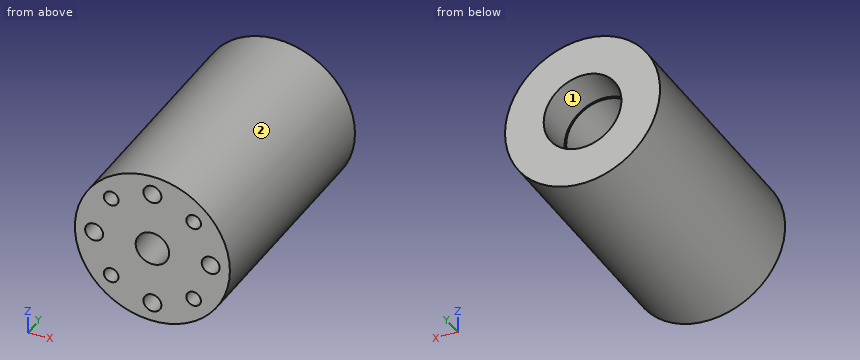
```python
from build123d import *

# Parameters (mm, degrees)
CUT_EXTRUDE2_START = -22.2
SKETCH4_R          = 1.1
SKETCH4_R_2        = 0.9
CUT_EXTRUDE2_DEPTH = 8


with BuildPart() as part:
    # Sketch1 → Revolve1 (revolve)
    with BuildSketch(Plane.XY):
        Polygon((4.762351203, 30), (4.762351203, 25), (4.559151203, 25), (2.05, 0), (9.5, -0.008522661), (9.5, 30), align=None)
    revolve(axis=Axis((0, 0, 0), (0, 1, 0)))

    # Sketch4 → Cut-Extrude2 (cut)
    with BuildSketch(Plane(origin=(0, 30, 0), x_dir=(1, 0, 0), z_dir=(0, 1, 0)).offset(CUT_EXTRUDE2_START)):
        with Locations(Location((0, 7.145, 0), (0, 0, 180))):
            Circle(SKETCH4_R)
        with Locations(Location((7.145, 0, 0), (0, 0, 180))):
            Circle(SKETCH4_R)
        with Locations(Location((0, -7.145, 0), (0, 0, 180))):
            Circle(SKETCH4_R)
        with Locations(Location((-7.145, 0, 0), (0, 0, 180))):
            Circle(SKETCH4_R)
        with Locations(Location((5.052277952, 5.052277952, 0), (0, 0, 180))):
            Circle(SKETCH4_R_2)
        with Locations(Location((5.052277952, -5.052277952, 0), (0, 0, 180))):
            Circle(SKETCH4_R_2)
        with Locations(Location((-5.052277952, -5.052277952, 0), (0, 0, 180))):
            Circle(SKETCH4_R_2)
        with Locations(Location((-5.052277952, 5.052277952, 0), (0, 0, 180))):
            Circle(SKETCH4_R_2)
    extrude(amount=-CUT_EXTRUDE2_DEPTH, mode=Mode.SUBTRACT)


solid = part.part
```
Check sheet for the modelled part. Datum: model origin and axes. Units: mm. Face numbers are marked on the shaded views. Round coordinates to 2 decimals unless told otherwise and drop trailing zeros. Loops run counter-clockwise (first coordinate to the right, second up) from the corner with the lowest first, then second, coordinate; pieces in that order, holes last. Notation, with made-up numbers: (-7.75, -9.5) -> (29.25, -9.5) arc R22 ccw to (29.25, 5.5) -> close; hole circle Ø4 at (4, -28.75). An arc over 180 degrees is marked (long way). Write item = value, one per line. Start each with the question number.
1) Sectioned sample at D-D, the plane y = 10. Record the cut outline in (x, z), plus the area to 3 significant figures.
2) Sectioned sample at C-C, the plane y = 20.5. Record the cut outline in (x, z) (1 decimal), plus the area to 3 significant figures.
3) Release check for a two-part mould opening along X. For the marked faces 1 and 2 record: released by +X, released by -X, zero draft, split by the parting line, or undercut.
4) Gauge pin test, flat ends, axial feed: pin 1 Ø2.5 at (x, z) = (-0.5, -7) entering from -Y; pin 2 Ø5 at (y, z) = (18, 3) entering from +X; pin 3 Ø1.6 at (x, z) = (5.05, 5.05) entering from -Y; pin 4 Ø5 at (x, y) = (-4.5, 24) entering from -Z. Record the tip position at first contact, or that the pin passes through.
5) Thickness scan on probe 1 along Z at (x, y) = (0, 5) (3 decimals); probe 2 along X at (y, z) = (6.25, 0) (3 decimals); probe 3 along Y at (x, z) = (-1, 6.25). Record the ranges inside material, lowest first.
6) Sectioned sample at B-B, the plane x = 0. Record the cut outline in (y, z) (3 decimals).
7) Sectioned sample at A-A, the plane z = 0. Record the cut outline in (x, y) (3 decimals).
Results are:
q1.outline = circle Ø19 at (0, 0); hole circle Ø6.11 at (0, 0)
q1.area = 254 mm^2
q2.outline = circle Ø19 at (0, 0); hole circle Ø8.2 at (0, 0)
q2.area = 231 mm^2
q3.face_1 = undercut
q3.face_2 = split by the parting line
q4.pin_1 = -0.01
q4.pin_2 = 9.49
q4.pin_3 = 7.8
q4.pin_4 = -9.29
q5.probe_1 = -9.5 to -8.245, -6.045 to -2.552, 2.552 to 6.045, 8.245 to 9.5
q5.probe_2 = -9.5 to -8.245, -6.045 to -2.677, 2.677 to 6.045, 8.245 to 9.5
q5.probe_3 = 0 to 30
q6.outline = (-0.009, -9.5) -> (30, -9.5) -> (30, -4.762) -> (25, -4.762) -> (25, -4.559) -> (0, -2.05) -> (-0.005, -6.045) -> (7.8, -6.045) -> (7.8, -8.245) -> (-0.007, -8.245) -> close; (-0.009, 9.5) -> (-0.007, 8.245) -> (7.8, 8.245) -> (7.8, 6.045) -> (-0.005, 6.045) -> (0, 2.05) -> (25, 4.559) -> (25, 4.762) -> (30, 4.762) -> (30, 9.5) -> close
q7.outline = (-9.5, -0.009) -> (-8.245, -0.007) -> (-8.245, 7.8) -> (-6.045, 7.8) -> (-6.045, -0.005) -> (-2.05, 0) -> (-4.559, 25) -> (-4.762, 25) -> (-4.762, 30) -> (-9.5, 30) -> close; (2.05, 0) -> (6.045, -0.005) -> (6.045, 7.8) -> (8.245, 7.8) -> (8.245, -0.007) -> (9.5, -0.009) -> (9.5, 30) -> (4.762, 30) -> (4.762, 25) -> (4.559, 25) -> close
